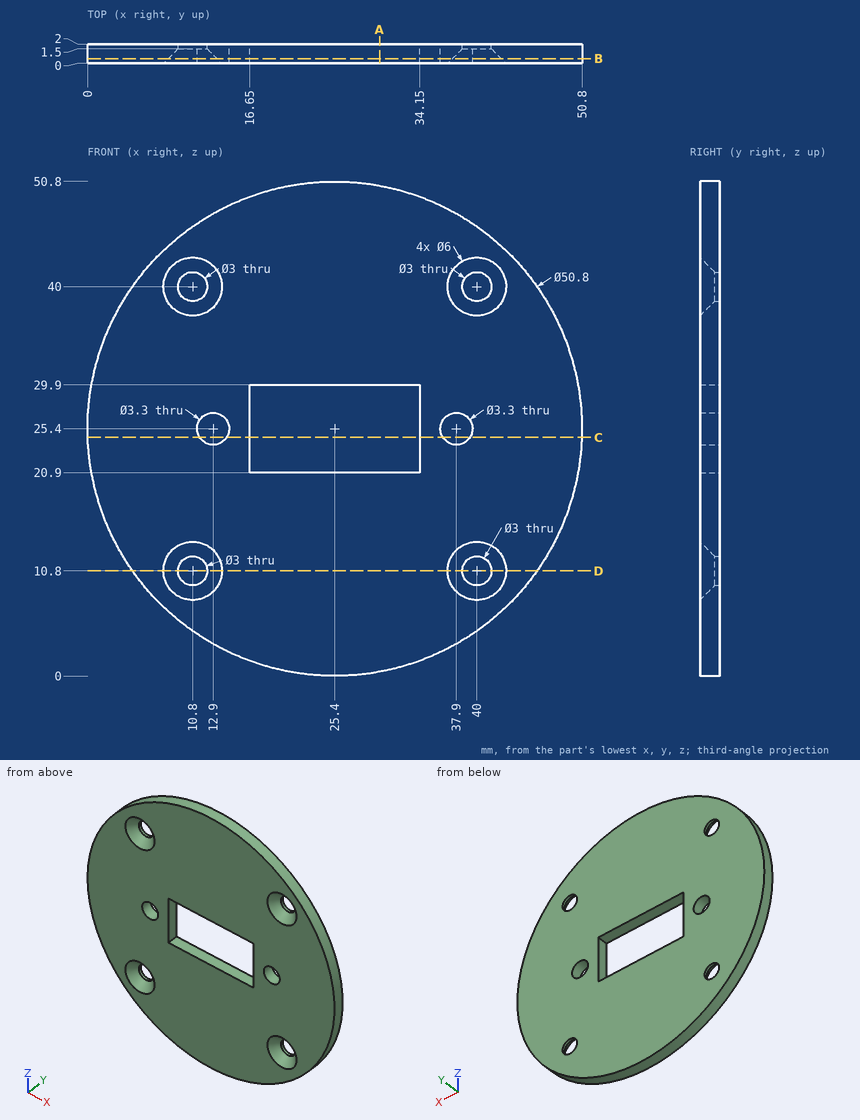
The drawing under review shows one solid part. Ordinate dimensions are in mm from its lowest x, y, z. Round coordinates to 2 decimals unless told otherwise and drop trailing zeros. Write each loop counter-clockwise with the first axis right and the second up, starting at its lowest first coordinate (ties: lowest second). Pieces come first, ordered by that corner, then holes. Notation, with made-up numbers: M 43.5,68.5 L 47.5,68.5 A11 cw 47.5,74.5 Z; hole C 40,53.5 d7. An arc over 180 degrees is marked long. One line per item, written item: value. Start each with the question number.
(1) Insertion check: pin 1 (2 mm diameter, centred on x = 6.5, z = 8.5, fed in from -Y); pin 2 (0.6 mm diameter, centred on x = 23.5, y = 0.5, fed in from +Z); pin 3 (1 mm diameter, centred on y = 1.5, z = 14.5, fed in from -X); pin 4 (0.6 mm diameter, centred on x = 27.5, y = 1, fed in from -Z). Each pin has a flat end and moves straight along its axis. Give the tip position at first contact, or say it passes through.
(2) We need section B-B (y = 0.5). Give the boundary of the cut face in (x, z).
(3) We need section C-C (z = 24.5). Give the boundary of the cut face in (x, y).
(4) Wall thickness on line 1 (X direction, y = 0.2, z = 25.5); line 2 (Z direction, x = 40, y = 1.7): over which ranges is each line inside the solid? List them lowest first.
(5) We need section A-A (x = 30). Give the boundary of the cut face in (y, z).
(6) We need section D-D (z = 10.8). Give the boundary of the cut face in (x, y), and give its area (3 significant figures).
Result:
1. pin 1: y = 0
1. pin 2: z = 50.75
1. pin 3: x = 2.23
1. pin 4: z = 0.06
2. outline: C 25.4,25.4 d50.8; hole C 10.8,10.8 d5; hole C 10.8,40 d5; hole C 12.9,25.4 d3.3; hole M 16.65,20.9 L 34.15,20.9 L 34.15,29.9 L 16.65,29.9 Z; hole C 37.9,25.4 d3.3; hole C 40,10.8 d5; hole C 40,40 d5
3. outline: M 0.02,0 L 11.52,0 L 11.52,2 L 0.02,2 Z; M 14.28,0 L 16.65,0 L 16.65,2 L 14.28,2 Z; M 34.15,0 L 36.52,0 L 36.52,2 L 34.15,2 Z; M 39.28,0 L 50.78,0 L 50.78,2 L 39.28,2 Z
4. line 1: 0 to 11.25, 14.55 to 16.65, 34.15 to 36.25, 39.55 to 50.8
4. line 2: 4.62 to 9.3, 12.3 to 38.5, 41.5 to 46.18
5. outline: M 0,0.42 L 2,0.42 L 2,20.9 L 0,20.9 Z; M 0,29.9 L 2,29.9 L 2,50.38 L 0,50.38 Z
6. outline: M 4.62,0 L 7.8,0 L 9.3,1.5 L 9.3,2 L 4.62,2 Z; M 12.3,1.5 L 13.8,0 L 37,0 L 38.5,1.5 L 38.5,2 L 12.3,2 Z; M 41.5,1.5 L 43,0 L 46.18,0 L 46.18,2 L 41.5,2 Z
6. area: 66.6 mm²
